from build123d import *

# Parameters (mm, degrees)
SKETCH1_W           = 60
SKETCH1_H           = 30
BOSS_EXTRUDE1_DEPTH = 28
SKETCH2_R           = 6
CUT_EXTRUDE1_DEPTH  = 28
SKETCH3_W           = 20
SKETCH3_H           = 20
BOSS_EXTRUDE3_DEPTH = 25
SKETCH5_W           = 12
SKETCH5_H           = 20
BOSS_EXTRUDE4_DEPTH = 15
SKETCH8_W           = 16
SKETCH8_H           = 20
BOSS_EXTRUDE5_DEPTH = 8


with BuildPart() as part:
    # Sketch1 → Boss-Extrude1 (new body)
    with BuildSketch(Plane.XY):
        with Locations((30, 15)):
            Rectangle(SKETCH1_W, SKETCH1_H)
    extrude(amount=BOSS_EXTRUDE1_DEPTH)

    # Sketch2 → Cut-Extrude1 (cut)
    with BuildSketch(Plane.XY.offset(28)):
        with Locations((44, 16)):
            Circle(SKETCH2_R)
    extrude(amount=-CUT_EXTRUDE1_DEPTH, mode=Mode.SUBTRACT)

    # Sketch3 → Boss-Extrude3 (add)
    with BuildSketch(Plane(origin=(0, 30, 0), x_dir=(1, 0, 0), z_dir=(0, 1, 0))):
        with Locations((10, -10)):
            Rectangle(SKETCH3_W, SKETCH3_H)
    extrude(amount=BOSS_EXTRUDE3_DEPTH)

    # Sketch5 → Boss-Extrude4 (add)
    with BuildSketch(Plane(origin=(0, 30, 0), x_dir=(1, 0, 0), z_dir=(0, 1, 0))):
        with Locations((26, -10)):
            Rectangle(SKETCH5_W, SKETCH5_H)
    extrude(amount=BOSS_EXTRUDE4_DEPTH)

    # Sketch8 → Boss-Extrude5 (add)
    with BuildSketch(Plane(origin=(0, 30, 0), x_dir=(1, 0, 0), z_dir=(0, 1, 0))):
        with Locations((40, -10)):
            Rectangle(SKETCH8_W, SKETCH8_H)
    extrude(amount=BOSS_EXTRUDE5_DEPTH)


solid = part.part
The listing builds one solid part. Answer for the finished solid, in the listing's coordinates (mm). A direction names the side the tool comes from. Give positions to 0.01 mm unless a question says otherwise; leave off trailing zeros. Loops run counter-clockwise (first coordinate to the right, second up) from the corner with the lowest first, then second, coordinate; pieces in that order, holes last. Notation, with made-up numbers: (64, 50) - (100, 50) arc R21 cw to (100, 81) - close; hole circle Ø3 at (89, 86.25). An arc over 180 degrees is marked (long way). Write each question's results on one line, items separated by ' | '.
1. Find section B-B, the plane y = 16. Write down the section's boundary in (x, z).
Resolved:
outline: (0, 0) - (38, 0) - (38, 28) - (0, 28) - close; (50, 0) - (60, 0) - (60, 28) - (50, 28) - close
2. Which of the six approach directions +Z, -Z, +X, -X, +Y, -Y give full straight-line access (tool end or side, diameter ignored) to faces 1 (the face through (18, 40, 20)), 2 (the face through (60, 15, 14)), 3 (the face through (40, 38, 10))?
Resolved:
face 1: +Z, +X, -X, +Y | face 2: +Z, -Z, +X, +Y, -Y | face 3: +Z, -Z, +X, +Y
3. Flat-ended cylindrical pins translate along their axes: P1, Ø8.5, axis at x = 37.5, z = 16, coming from the +Y side; P2, Ø3, axis at y = 33.5, z = 13, coming from the +X side; P3, Ø3.5, axis at y = 40, z = 12.5, coming from the +X side. Find the tip coordinate at first contact, or state that the pin passes through.
Resolved:
P1: stops at y = 38 | P2: stops at x = 48 | P3: stops at x = 32
4. Find section C-C, the plane z = 12.75. Write down the section's boundary in (x, y).
Resolved:
outline: (0, 0) - (60, 0) - (60, 30) - (48, 30) - (48, 38) - (32, 38) - (32, 45) - (20, 45) - (20, 55) - (0, 55) - close; hole circle Ø12 at (44, 16)
5. For a pull along X with two mould halves and no side action, classify faces 4 (the face through (38, 16, 14)), 5 (the face through (23, 21, 0)), 6 (the face through (20, 50, 10)), 7 (the face through (0, 27, 11)) as +X half, -X half, draft (parallel to the pull), parting line (faces both ways), or undercut.
Resolved:
face 4: undercut | face 5: draft | face 6: +X half | face 7: -X half
6. Find section A-A, the plane x = 44. Write down the section's boundary in (y, z), then the cut area to 3 significant figures.
Resolved:
outline: (0, 0) - (10, 0) - (10, 28) - (0, 28) - close; (22, 0) - (38, 0) - (38, 20) - (30, 20) - (30, 28) - (22, 28) - close | area: 664 mm^2
7. Consider probe 1 along Y at (x, z) = (44, 19.5); probe 2 along Z at (x, y) = (26.5, 44); probe 3 along Y at (x, z) = (52, 10.75). Determine where each line is inside the solid, lowest interval first. Write a range as from..to.
Resolved:
probe 1: y = 0..10, 22..38 | probe 2: z = 0..20 | probe 3: y = 0..30
8. Find section D-D, the plane x = 30. Write down the section's boundary in (y, z).
Resolved:
outline: (0, 0) - (45, 0) - (45, 20) - (30, 20) - (30, 28) - (0, 28) - close
